Read the model definition and answer for the solid it produces. Units are mm, in the model's axes. Coordinates: 2 decimals unless noted, no trailing zeros. Write each loop counter-clockwise with the first axis right and the second up, starting at its lowest first coordinate (ties: lowest second). Pieces come first, ordered by that corner, then holes. Notation, with made-up numbers: (68, -29.75) -> (115, -29.75) arc R25 cw to (115, -15.75) -> close; hole circle Ø4 at (30, 10.25). An arc over 180 degrees is marked (long way). One line per item, written item: value. Start each with the question number.
1. Consider line 1 along Z through (x, y) = (0.2, -0.75) (3 decimals); line 2 along Y through (x, z) = (0.7, 10.75); line 3 along X through (y, z) = (-0.25, 10.5) (3 decimals). Determine where each line is inside the solid, lowest interval first.
2. Find section B-B, the plane z = 5. Write down the section's boundary in (x, y) (3 decimals).
3. Find section A-A, the plane y = -1.25. Write down the section's boundary in (x, z) (3 decimals).
4. Given P1, Ø0.8, axis at y = -1, z = 7.5, coming from the +X side (3 decimals); P2, Ø1.5, axis at x = 0.5, y = -1, coming from the +Z side (3 decimals); P3, Ø0.6, axis at y = 6, z = 12.5, coming from the -X side (3 decimals), each flat-ended and moving along its own axis, determine where each tip first touches the part or whether it passes through.
5. For a pull along Z with two mould halves and no side action, classify faces 1 (the flat face through (0, 2.3, 11)), 2 (the flat face through (0, 1, 19.07)), 3 (the flat face through (0, 1, 3.83)) as pulls with the +Z half, pulls with the -Z half, needs draft (parallel to the pull), parting line crosses it, or undercut.
```python
from build123d import *

# Parameters (mm, degrees)
CROQUIS1_W               = 2.54
CROQUIS1_H               = 15.24
SALIENTE_EXTRUIR1_DEPTH  = 2.3
CORTAR_EXTRUIR4_DEPTH    = 2.3
CORTAR_EXTRUIR5_DEPTH    = 2.3
CORTAR_EXTRUIR6_DEPTH    = 2.3
CORTAR_EXTRUIR7_DEPTH    = 2.3
CORTAR_EXTRUIR8_DEPTH    = 2.3
CORTAR_EXTRUIR9_DEPTH    = 2.3
CORTAR_EXTRUIR10_DEPTH   = 2.3
CORTAR_EXTRUIR13_DEPTH   = 2.3
CORTAR_EXTRUIR14_DEPTH   = 2.3
CORTAR_EXTRUIR15_DEPTH   = 2.3
CORTAR_EXTRUIR16_DEPTH   = 2.3
CORTAR_EXTRUIR17_DEPTH   = 2.3
CORTAR_EXTRUIR18_DEPTH   = 2.3
CORTAR_EXTRUIR19_DEPTH   = 2.3
CROQUIS27_W              = 0.75
CROQUIS27_H              = 0.75
SALIENTE_EXTRUIR5_DEPTH  = 6.2
CROQUIS28_W              = 0.75
CROQUIS28_H              = 0.75
SALIENTE_EXTRUIR6_DEPTH  = 6.2
CROQUIS29_W              = 0.75
CROQUIS29_H              = 0.75
SALIENTE_EXTRUIR7_DEPTH  = 6.2
CROQUIS30_W              = 0.75
CROQUIS30_H              = 0.75
SALIENTE_EXTRUIR8_DEPTH  = 6.2
CROQUIS31_W              = 0.75
CROQUIS31_H              = 0.75
SALIENTE_EXTRUIR9_DEPTH  = 6.2
CROQUIS32_W              = 0.75
CROQUIS32_H              = 0.75
SALIENTE_EXTRUIR10_DEPTH = 6.2
CROQUIS38_W              = 0.75
CROQUIS38_H              = 0.75
SALIENTE_EXTRUIR16_DEPTH = 3.25
CROQUIS39_W              = 0.75
CROQUIS39_H              = 0.75
SALIENTE_EXTRUIR17_DEPTH = 3.25
CROQUIS40_W              = 0.75
CROQUIS40_H              = 0.75
SALIENTE_EXTRUIR18_DEPTH = 3.25
CROQUIS41_W              = 0.75
CROQUIS41_H              = 0.75
SALIENTE_EXTRUIR19_DEPTH = 3.25
CROQUIS42_W              = 0.75
CROQUIS42_H              = 0.75
SALIENTE_EXTRUIR20_DEPTH = 3.25
CROQUIS43_W              = 0.75
CROQUIS43_H              = 0.75
SALIENTE_EXTRUIR21_DEPTH = 3.25


with BuildPart() as part:
    # Croquis1 → Saliente-Extruir1 (new body)
    with BuildSketch(Plane(origin=(0, 2.3, 0), x_dir=(1, 0, 0), z_dir=(0, 1, 0))):
        with Locations((0, -11.45)):
            Rectangle(CROQUIS1_W, CROQUIS1_H)
    extrude(amount=-SALIENTE_EXTRUIR1_DEPTH)

    # Croquis5 → Cortar-Extruir4 (cut)
    with BuildSketch(Plane.XZ):
        with BuildLine():
            Line((1.27, 18.55), (1.27, 19.55))
            ThreePointArc((1.27, 19.55), (1.123553391, 19.196446609), (0.77, 19.05))
            ThreePointArc((0.77, 19.05), (1.123553391, 18.903553391), (1.27, 18.55))
        make_face()
    extrude(amount=-CORTAR_EXTRUIR4_DEPTH, mode=Mode.SUBTRACT)

    # Croquis6 → Cortar-Extruir5 (cut)
    with BuildSketch(Plane.XZ):
        with BuildLine():
            Line((1.27, 16.01), (1.27, 17.01))
            ThreePointArc((1.27, 17.01), (1.123553391, 16.656446609), (0.77, 16.51))
            ThreePointArc((0.77, 16.51), (1.123553391, 16.363553391), (1.27, 16.01))
        make_face()
    extrude(amount=-CORTAR_EXTRUIR5_DEPTH, mode=Mode.SUBTRACT)

    # Croquis7 → Cortar-Extruir6 (cut)
    with BuildSketch(Plane.XZ):
        with BuildLine():
            Line((1.27, 13.47), (1.27, 14.47))
            ThreePointArc((1.27, 14.47), (1.123553391, 14.116446609), (0.77, 13.97))
            ThreePointArc((0.77, 13.97), (1.123553391, 13.823553391), (1.27, 13.47))
        make_face()
    extrude(amount=-CORTAR_EXTRUIR6_DEPTH, mode=Mode.SUBTRACT)

    # Croquis8 → Cortar-Extruir7 (cut)
    with BuildSketch(Plane.XZ):
        with BuildLine():
            Line((1.27, 10.93), (1.27, 11.93))
            ThreePointArc((1.27, 11.93), (1.123553391, 11.576446609), (0.77, 11.43))
            ThreePointArc((0.77, 11.43), (1.123553391, 11.283553391), (1.27, 10.93))
        make_face()
    extrude(amount=-CORTAR_EXTRUIR7_DEPTH, mode=Mode.SUBTRACT)

    # Croquis9 → Cortar-Extruir8 (cut)
    with BuildSketch(Plane.XZ):
        with BuildLine():
            Line((1.27, 8.39), (1.27, 9.39))
            ThreePointArc((1.27, 9.39), (1.123553391, 9.036446609), (0.77, 8.89))
            ThreePointArc((0.77, 8.89), (1.123553391, 8.743553391), (1.27, 8.39))
        make_face()
    extrude(amount=-CORTAR_EXTRUIR8_DEPTH, mode=Mode.SUBTRACT)

    # Croquis10 → Cortar-Extruir9 (cut)
    with BuildSketch(Plane.XZ):
        with BuildLine():
            Line((1.27, 5.85), (1.27, 6.85))
            ThreePointArc((1.27, 6.85), (1.123553391, 6.496446609), (0.77, 6.35))
            ThreePointArc((0.77, 6.35), (1.123553391, 6.203553391), (1.27, 5.85))
        make_face()
    extrude(amount=-CORTAR_EXTRUIR9_DEPTH, mode=Mode.SUBTRACT)

    # Croquis11 → Cortar-Extruir10 (cut)
    with BuildSketch(Plane.XZ):
        with BuildLine():
            Line((1.27, 3.31), (1.27, 4.31))
            ThreePointArc((1.27, 4.31), (1.123553391, 3.956446609), (0.77, 3.81))
            ThreePointArc((0.77, 3.81), (1.123553391, 3.663553391), (1.27, 3.31))
        make_face()
    extrude(amount=-CORTAR_EXTRUIR10_DEPTH, mode=Mode.SUBTRACT)

    # Croquis14 → Cortar-Extruir13 (cut)
    with BuildSketch(Plane.XZ):
        with BuildLine():
            Line((-1.27, 4.31), (-1.27, 3.31))
            ThreePointArc((-1.27, 3.31), (-1.123553391, 3.663553391), (-0.77, 3.81))
            ThreePointArc((-0.77, 3.81), (-1.123553391, 3.956446609), (-1.27, 4.31))
        make_face()
    extrude(amount=-CORTAR_EXTRUIR13_DEPTH, mode=Mode.SUBTRACT)

    # Croquis15 → Cortar-Extruir14 (cut)
    with BuildSketch(Plane.XZ):
        with BuildLine():
            Line((-1.27, 6.85), (-1.27, 5.85))
            ThreePointArc((-1.27, 5.85), (-1.123553391, 6.203553391), (-0.77, 6.35))
            ThreePointArc((-0.77, 6.35), (-1.123553391, 6.496446609), (-1.27, 6.85))
        make_face()
    extrude(amount=-CORTAR_EXTRUIR14_DEPTH, mode=Mode.SUBTRACT)

    # Croquis16 → Cortar-Extruir15 (cut)
    with BuildSketch(Plane.XZ):
        with BuildLine():
            Line((-1.27, 9.39), (-1.27, 8.39))
            ThreePointArc((-1.27, 8.39), (-1.123553391, 8.743553391), (-0.77, 8.89))
            ThreePointArc((-0.77, 8.89), (-1.123553391, 9.036446609), (-1.27, 9.39))
        make_face()
    extrude(amount=-CORTAR_EXTRUIR15_DEPTH, mode=Mode.SUBTRACT)

    # Croquis17 → Cortar-Extruir16 (cut)
    with BuildSketch(Plane.XZ):
        with BuildLine():
            Line((-1.27, 11.93), (-1.27, 10.93))
            ThreePointArc((-1.27, 10.93), (-1.123553391, 11.283553391), (-0.77, 11.43))
            ThreePointArc((-0.77, 11.43), (-1.123553391, 11.576446609), (-1.27, 11.93))
        make_face()
    extrude(amount=-CORTAR_EXTRUIR16_DEPTH, mode=Mode.SUBTRACT)

    # Croquis18 → Cortar-Extruir17 (cut)
    with BuildSketch(Plane.XZ):
        with BuildLine():
            Line((-1.27, 14.47), (-1.27, 13.47))
            ThreePointArc((-1.27, 13.47), (-1.123553391, 13.823553391), (-0.77, 13.97))
            ThreePointArc((-0.77, 13.97), (-1.123553391, 14.116446609), (-1.27, 14.47))
        make_face()
    extrude(amount=-CORTAR_EXTRUIR17_DEPTH, mode=Mode.SUBTRACT)

    # Croquis19 → Cortar-Extruir18 (cut)
    with BuildSketch(Plane.XZ):
        with BuildLine():
            Line((-1.27, 17.01), (-1.27, 16.01))
            ThreePointArc((-1.27, 16.01), (-1.123553391, 16.363553391), (-0.77, 16.51))
            ThreePointArc((-0.77, 16.51), (-1.123553391, 16.656446609), (-1.27, 17.01))
        make_face()
    extrude(amount=-CORTAR_EXTRUIR18_DEPTH, mode=Mode.SUBTRACT)

    # Croquis20 → Cortar-Extruir19 (cut)
    with BuildSketch(Plane.XZ):
        with BuildLine():
            Line((-1.27, 19.55), (-1.27, 18.55))
            ThreePointArc((-1.27, 18.55), (-1.123553391, 18.903553391), (-0.77, 19.05))
            ThreePointArc((-0.77, 19.05), (-1.123553391, 19.196446609), (-1.27, 19.55))
        make_face()
    extrude(amount=-CORTAR_EXTRUIR19_DEPTH, mode=Mode.SUBTRACT)

    # Croquis27 → Saliente-Extruir5 (add)
    with BuildSketch(Plane(origin=(0, 2.3, 0), x_dir=(-1, 0, 0), z_dir=(0, 1, 0))):
        with Locations((0, 5.08)):
            Rectangle(CROQUIS27_W, CROQUIS27_H)
    extrude(amount=SALIENTE_EXTRUIR5_DEPTH)

    # Croquis28 → Saliente-Extruir6 (add)
    with BuildSketch(Plane(origin=(0, 2.3, 0), x_dir=(-1, 0, 0), z_dir=(0, 1, 0))):
        with Locations((0, 7.62)):
            Rectangle(CROQUIS28_W, CROQUIS28_H)
    extrude(amount=SALIENTE_EXTRUIR6_DEPTH)

    # Croquis29 → Saliente-Extruir7 (add)
    with BuildSketch(Plane(origin=(0, 2.3, 0), x_dir=(-1, 0, 0), z_dir=(0, 1, 0))):
        with Locations((0, 10.16)):
            Rectangle(CROQUIS29_W, CROQUIS29_H)
    extrude(amount=SALIENTE_EXTRUIR7_DEPTH)

    # Croquis30 → Saliente-Extruir8 (add)
    with BuildSketch(Plane(origin=(0, 2.3, 0), x_dir=(-1, 0, 0), z_dir=(0, 1, 0))):
        with Locations((0, 12.7)):
            Rectangle(CROQUIS30_W, CROQUIS30_H)
    extrude(amount=SALIENTE_EXTRUIR8_DEPTH)

    # Croquis31 → Saliente-Extruir9 (add)
    with BuildSketch(Plane(origin=(0, 2.3, 0), x_dir=(-1, 0, 0), z_dir=(0, 1, 0))):
        with Locations((0, 15.24)):
            Rectangle(CROQUIS31_W, CROQUIS31_H)
    extrude(amount=SALIENTE_EXTRUIR9_DEPTH)

    # Croquis32 → Saliente-Extruir10 (add)
    with BuildSketch(Plane(origin=(0, 2.3, 0), x_dir=(-1, 0, 0), z_dir=(0, 1, 0))):
        with Locations((0, 17.78)):
            Rectangle(CROQUIS32_W, CROQUIS32_H)
    extrude(amount=SALIENTE_EXTRUIR10_DEPTH)

    # Croquis38 → Saliente-Extruir16 (add)
    with BuildSketch(Plane.XZ):
        with Locations((0, 5.08)):
            Rectangle(CROQUIS38_W, CROQUIS38_H)
    extrude(amount=SALIENTE_EXTRUIR16_DEPTH)

    # Croquis39 → Saliente-Extruir17 (add)
    with BuildSketch(Plane.XZ):
        with Locations((0, 7.62)):
            Rectangle(CROQUIS39_W, CROQUIS39_H)
    extrude(amount=SALIENTE_EXTRUIR17_DEPTH)

    # Croquis40 → Saliente-Extruir18 (add)
    with BuildSketch(Plane.XZ):
        with Locations((0, 10.16)):
            Rectangle(CROQUIS40_W, CROQUIS40_H)
    extrude(amount=SALIENTE_EXTRUIR18_DEPTH)

    # Croquis41 → Saliente-Extruir19 (add)
    with BuildSketch(Plane.XZ):
        with Locations((0, 12.7)):
            Rectangle(CROQUIS41_W, CROQUIS41_H)
    extrude(amount=SALIENTE_EXTRUIR19_DEPTH)

    # Croquis42 → Saliente-Extruir20 (add)
    with BuildSketch(Plane.XZ):
        with Locations((0, 15.24)):
            Rectangle(CROQUIS42_W, CROQUIS42_H)
    extrude(amount=SALIENTE_EXTRUIR20_DEPTH)

    # Croquis43 → Saliente-Extruir21 (add)
    with BuildSketch(Plane.XZ):
        with Locations((0, 17.78)):
            Rectangle(CROQUIS43_W, CROQUIS43_H)
    extrude(amount=SALIENTE_EXTRUIR21_DEPTH)


solid = part.part
```
Answer block:
1. line 1: z = 4.705 to 5.455, 7.245 to 7.995, 9.785 to 10.535, 12.325 to 13.075, 14.865 to 15.615, 17.405 to 18.155
1. line 2: y = 0 to 2.3
1. line 3: x = -0.375 to 0.375
2. outline: (-1.27, 0) -> (-0.375, 0) -> (-0.375, -3.25) -> (0.375, -3.25) -> (0.375, 0) -> (1.27, 0) -> (1.27, 2.3) -> (0.375, 2.3) -> (0.375, 8.5) -> (-0.375, 8.5) -> (-0.375, 2.3) -> (-1.27, 2.3) -> close
3. outline: (-0.375, 4.705) -> (0.375, 4.705) -> (0.375, 5.455) -> (-0.375, 5.455) -> close; (-0.375, 7.245) -> (0.375, 7.245) -> (0.375, 7.995) -> (-0.375, 7.995) -> close; (-0.375, 9.785) -> (0.375, 9.785) -> (0.375, 10.535) -> (-0.375, 10.535) -> close; (-0.375, 12.325) -> (0.375, 12.325) -> (0.375, 13.075) -> (-0.375, 13.075) -> close; (-0.375, 14.865) -> (0.375, 14.865) -> (0.375, 15.615) -> (-0.375, 15.615) -> close; (-0.375, 17.405) -> (0.375, 17.405) -> (0.375, 18.155) -> (-0.375, 18.155) -> close
4. P1: stops at x = 0.375
4. P2: stops at z = 18.155
4. P3: stops at x = -0.375
5. face 1: undercut
5. face 2: pulls with the +Z half
5. face 3: pulls with the -Z half
